Autodesk Inventor part; units mm, degrees
ref_plane "Work Plane1" through (0, 0, 20) normal (0, 0, 1) x (1, 0, 0)
ref_plane "YZ Plane" through (0, 0, 0) normal (1, 0, 0) x (0, 1, 0)
ref_plane "XZ Plane" through (0, 0, 0) normal (0, 1, 0) x (-1, 0, 0)
sketch "Sketch1" plane through (0, 0, 0) normal (0, 0, 1) x (1, 0, 0)
  line L0 (-152.5, -50) -> (152.5, -50)
  line L1 (152.5, -50) -> (152.5, 50)
  line L2 (152.5, 50) -> (-152.5, 50)
  line L3 (-152.5, 50) -> (-152.5, -50)
  line L4 (-152.5, -50) -> (152.5, 50) construction
  line L5 (152.5, -50) -> (-152.5, 50) construction
  point P0 (0, 0)
  dimension "d0" = 305
  dimension "d1" = 100
extrude "Extrusion1" add sketch "Sketch1" along normal blind 10
sketch "Sketch4" plane through (152.5, -50, 0) normal (1, 0, 0) x (0, 0, -1)
  circle A0 centre (-80, 0) radius 50 construction
  line L0 (0, 0) -> (-10, 0)
  line L1 (0, 0) -> (-48.75, -39.0312)
  line L2 (-10, 0) -> (-10, 100)
  line L3 (-10, 100) -> (-105.6226, 42.9358)
  arc A1 (-105.6226, 42.9358) -> (-48.75, -39.0312) centre (-80, 0) ccw
  line L4 (0, 0) -> (-10, 0)
  line L5 (-10, 100) -> (-10, 0)
  dimension "d8" = 100
  dimension "d20" = 80
extrude "Extrusion3" add sketch "Sketch4" against normal blind 305
ref_plane "Work Plane1" through (0, 0, 20) normal (0, 0, 1) x (1, 0, 0)
sketch "Sketch5" plane through (0, 0, 20) normal (0, 0, 1) x (1, 0, 0)
  line L0 (152.5, 50) -> (-152.5, 50)
  line L1 (152.5, -100) -> (-152.5, -100)
  line L2 (-142.5, 50) -> (142.5, 50)
  line L3 (142.5, 50) -> (142.5, -100)
  line L4 (142.5, -100) -> (-142.5, -100)
  line L5 (-142.5, -100) -> (-142.5, 50)
  line L6 (-152.5, 50) -> (-152.5, -50)
  line L7 (152.5, -50) -> (152.5, 50)
  point P0 (0, 0)
  dimension "d16" = 10
  dimension "d17" = 10
extrude "Extrusion4" cut sketch "Sketch5" along normal through all
sketch "Sketch9" plane through (152.5, -50, 0) normal (1, 0, 0) x (0, 0, -1)
  arc A0 (-105.6226, 42.9358) -> (-48.75, -39.0312) centre (-80, 0) ccw
  circle A1 centre (-80, 0) radius 2.5
  point P0 (0, 50)
  dimension "d28" = 5
extrude "Extrusion8" cut sketch "Sketch9" against normal through all
sketch "Sketch11" plane through (0, 0, 20) normal (0, 0, 1) x (1, 0, 0)
  circle A0 centre (30, 0) radius 2.5
  circle A1 centre (15, 25.9808) radius 2.5
  circle A2 centre (-15, 25.9808) radius 2.5
  circle A3 centre (-30, 0) radius 2.5
  circle A4 centre (-15, -25.9808) radius 2.5
  circle A5 centre (15, -25.9808) radius 2.5
  circle A6 centre (0, 0) radius 15
  dimension "d33" = 5
  dimension "d34" = 30
  dimension "d37" = 360
  dimension "d41" = 30
extrude "Extrusion10" cut sketch "Sketch11" against normal through all contours A0 | A1 | A2 | A3 | A4 | A5
sketch "Sketch14" plane through (-142.5, -66.0128, 20) normal (1, 0, 0) x (0, 0, -1)
  circle A0 centre (-60, 16.0128) radius 2.5
  circle A1 centre (-60, 22.3628) radius 1.5
  circle A2 centre (-66.35, 16.0128) radius 1.5
  circle A3 centre (-60, 9.6628) radius 1.5
  circle A4 centre (-53.65, 16.0128) radius 1.5
  point P0 (20, 66.0128)
  dimension "d49" = 3
  dimension "d50" = 6.35
  dimension "d53" = 360
extrude "Extrusion12" cut sketch "Sketch14" along normal through all both and the other way through all contours A1 | A2 | A3 | A4
sketch "Sketch15" plane through (0, 0, 20) normal (0, 0, 1) x (1, 0, 0)
  line L0 (152.5, 50) -> (-152.5, 50)
  line L1 (-152.5, -7.0642) -> (-152.5, -100)
  line L2 (0, 50) -> (-152.5, 50)
  line L3 (-152.5, 50) -> (-152.5, -100)
  line L4 (-152.5, -100) -> (0, -100)
  line L5 (0, -100) -> (0, 50)
  point P0 (0, 0)
  point P1 (-152.5, -89.0312)
extrude "Extrusion13" cut sketch "Sketch15" along normal through all both and the other way through all
sketch "Sketch16" plane through (152.5, -50, 0) normal (1, 0, 0) x (0, 0, -1)
  circle A0 centre (-80, 0) radius 2.5
  circle A1 centre (-80, 0) radius 12.5
  circle A2 centre (-80, -6.35) radius 1.5 construction
  circle A3 centre (-80, 6.35) radius 1.5 construction
  circle A4 centre (-86.35, 0) radius 1.5 construction
  circle A5 centre (-73.65, 0) radius 1.5 construction
  circle A6 centre (-80, 0) radius 2.5
  line L0 (0, 0) -> (0, 100)
  line L1 (0, 100) -> (-10, 100)
  line L2 (-10, 100) -> (-105.6226, 42.9358)
  arc A7 (-105.6226, 42.9358) -> (-48.75, -39.0312) centre (-80, 0) ccw
  line L3 (-48.75, -39.0312) -> (0, 0)
  point P0 (0, 50)
  dimension "d59" = 25
extrude "Extrusion14" add sketch "Sketch16" along normal blind 10 contours L3 A7 L2 L1 L0
sketch "Sketch17" plane through (0, 0, 20) normal (0, 0, 1) x (1, 0, 0)
  circle A0 centre (30, 0) radius 2.5
  circle A1 centre (30, 0) radius 6.5
  circle A2 centre (15, 25.9808) radius 6.5
  circle A3 centre (-15, 25.9808) radius 6.5
  circle A4 centre (-30, 0) radius 6.5
  circle A5 centre (-15, -25.9808) radius 6.5
  circle A6 centre (15, -25.9808) radius 6.5
  point P0 (0, 0)
  dimension "d62" = 13
  dimension "d65" = 360
extrude "Extrusion15" cut sketch "Sketch17" against normal blind 5 contours A0 | A1 | A2 | A3 | A4 | A5 | A6
properties part number "HA004"
Build history of the part. All positions in model axes, mm. A direction names the side the tool comes from. Give positions to 0.01 mm unless a question says otherwise; leave off trailing zeros. Loops run counter-clockwise (first coordinate to the right, second up) from the corner with the lowest first, then second, coordinate; pieces in that order, holes last.
1) Band-saw the part on B-B on y = 0. List the corners of the cut face in (x, z), then the cut area to 3 significant figures.
Values follow:
outline: (0, 0) - (27.5, 0) - (27.5, 15) - (23.5, 15) - (23.5, 20) - (0, 20) - close; (32.5, 0) - (162.5, 0) - (162.5, 93.79) - (142.5, 93.79) - (142.5, 20) - (36.5, 20) - (36.5, 15) - (32.5, 15) - close
area: 4,590 mm2
2) Band-saw the part on C-C on x = 55.5. List the corners of the cut face in (y, z), then the cut area to 3 significant figures.
Values follow:
outline: (-66.01, 20) - (-50, 0) - (50, 0) - (50, 10) - (44.03, 20) - close
area: 2,130 mm2
3) Band-saw the part on D-D on z = 45. List the corners of the cut face in (x, y), then the cut area to 3 significant figures.
Values follow:
outline: (142.5, -86.03) - (162.5, -86.03) - (162.5, 29.11) - (142.5, 29.11) - close
area: 2,300 mm2
4) Probe line 1 along Y through (x, z) = (15, 18); line 2 along Y through (x, z) = (148, 80); line 3 along Y through (x, z) = (15, 17). List the from-to ranges inside material, lowest first.
Values follow:
line 1: y = -64.41 to -32.48, -19.48 to 19.48, 32.48 to 45.23
line 2: y = -100 to -57.85, -54.85 to -52.5, -47.5 to -45.15, -42.15 to 8.23
line 3: y = -63.61 to -32.48, -19.48 to 19.48, 32.48 to 45.82
5) Two-plate mould, pull along Y, no slides. Class faces 1 (the face through (0, -9, 10)), 2 (the face through (8.506, -25.695, 17.535)), 3 (the face through (8.506, 26.267, 17.535)), 4 (the face through (152.36, -79.438, 120.415)): released by +Y, released by -Y, zero draft, split by the parting line, or undercut.
Values follow:
face 1: zero draft
face 2: undercut
face 3: undercut
face 4: split by the parting line
6) Band-saw the part on A-A on x = 30. List the corners of the cut face in (y, z), then the cut area to 3 significant figures.
Values follow:
outline: (-66.01, 20) - (-50, 0) - (-2.5, 0) - (-2.5, 15) - (-6.5, 15) - (-6.5, 20) - close; (2.5, 0) - (50, 0) - (50, 10) - (44.03, 20) - (6.5, 20) - (6.5, 15) - (2.5, 15) - close
area: 1,990 mm2
7) 3-axis set-ups, long thin cutter, end or side, ignore diameter. For faces 5 (the face through (157.43, -45.212, 68.453)), 6 (the face through (80, -1, 0)), 7 (the face through (70, -10, 20)), 8 (the face through (23.506, 0.286, 17.535)): which of +Z, -Z, +X, -X, +Y, -Y reach the whole face in a straight line?
Values follow:
face 5: +X
face 6: -Z, +X, -X, +Y, -Y
face 7: +Z, -X, +Y, -Y
face 8: +Z
8) Drop flat-ended pins along their axis: P1, Ø1.5, axis at x = 52.5, y = -49, coming from the +Z side; P2, Ø5, axis at y = -50, z = 86.35, coming from the -X side; P3, Ø6.5, axis at x = 12.5, y = 26, coming from the +Z side. Give the stop position or say it passes through.
Values follow:
P1: stops at z = 20
P2: stops at x = 142.5
P3: stops at z = 15
